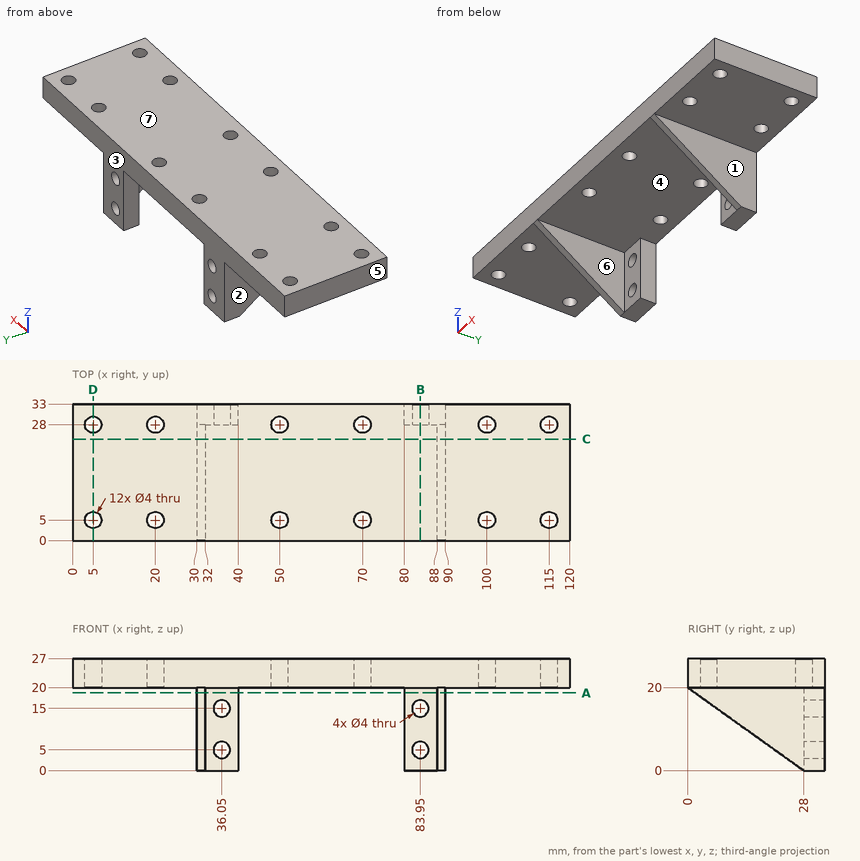
Here's the drawing with two shaded views (mm, measured from the low corner). I have some questions. A direction names the side the tool comes from. Give positions to 0.01 mm unless a question says otherwise; leave off trailing zeros. Write each loop counter-clockwise with the first axis right and the second up, starting at its lowest first coordinate (ties: lowest second). Pieces come first, ordered by that corner, then holes. Notation, with made-up numbers: (-39, 54.25) -> (18, 54.25) arc R10 cw to (18, 62.25) -> close; hole circle Ø10 at (88.25, 67). An arc over 180 degrees is marked (long way). Use one line per item in the form item = value. Start each with the question number.
1. Imagine slicing it at C-C on y = 24.5. List the corners of the cut face in (x, z) for me.
2. Imagine slicing it at A-A on z = 18.75. List the corners of the cut face in (x, y) for me, plus the area to 3 significant figures.
3. Imagine slicing it at D-D on x = 5. List the corners of the cut face in (y, z) for me.
4. Will these pins go through, and if not, where does the flat tip stop? pin 1 Ø10 at (y, z) = (24.5, 12) entering from +X; pin 2 Ø2.5 at (x, z) = (83.95, 5) entering from -Y; pin 3 Ø9 at (x, y) = (110, 14) entering from -Z; pin 4 Ø4 at (y, z) = (30.5, 13) entering from -X.
5. Thinking about a two-plate mould opening in X: for the marked faces 4, 5, 6 and 7, which applies, +X half, -X half, draft (parallel to the pull), parting line (faces both ways), or undercut?
6. Imagine slicing it at B-B on x = 83.95. List the corners of the cut face in (y, z) for me.
7. If I drill on L1, parallel to Y at x = 100, z = 25; L2, parallel to X at y = 29.4, z = 5; L3, parallel to Z at x = 59.5, y = 20.5, over which ranges is the centre line in solid material (lowest first)?
8. On a 3-axis mill with a long thin cutter (end or side, diameter ignored), from which of +Z, -Z, +X, -X, +Y, -Y can I reach the whole of each face in a straight line? I mean the marked faces 1, 2 and 3. Say none if no direction works.
Entries:
q1.outline = (0, 20) -> (30, 20) -> (30, 2.5) -> (32, 2.5) -> (32, 20) -> (88, 20) -> (88, 2.5) -> (90, 2.5) -> (90, 20) -> (120, 20) -> (120, 27) -> (0, 27) -> close
q2.outline = (30, 1.75) -> (32, 1.75) -> (32, 28) -> (40, 28) -> (40, 33) -> (30, 33) -> close; (80, 28) -> (88, 28) -> (88, 1.75) -> (90, 1.75) -> (90, 33) -> (80, 33) -> close
q2.area = 205 mm²
q3.outline = (0, 20) -> (3, 20) -> (3, 27) -> (0, 27) -> close; (7, 20) -> (26, 20) -> (26, 27) -> (7, 27) -> close; (30, 20) -> (33, 20) -> (33, 27) -> (30, 27) -> close
q4.pin_1 = 90
q4.pin_2 = through
q4.pin_3 = 20
q4.pin_4 = 30
q5.face_4 = undercut
q5.face_5 = -X half
q5.face_6 = undercut
q5.face_7 = draft
q6.outline = (0, 20) -> (28, 20) -> (28, 17) -> (33, 17) -> (33, 27) -> (0, 27) -> close; (28, 0) -> (33, 0) -> (33, 3) -> (28, 3) -> close; (28, 7) -> (33, 7) -> (33, 13) -> (28, 13) -> close
q7.L1 = 0 to 3, 7 to 26, 30 to 33
q7.L2 = 30 to 34.05, 38.05 to 40, 80 to 81.95, 85.95 to 90
q7.L3 = 20 to 27
q8.face_1 = -Z, +X, +Y, -Y
q8.face_2 = -Z, -X, +Y, -Y
q8.face_3 = +Z, -Z, +X, -X, +Y
